Here's how the part is built. I have some questions about the finished solid (model axes, mm). Coordinates: 2 decimals unless noted, no trailing zeros. Loops run counter-clockwise (first coordinate to the right, second up) from the corner with the lowest first, then second, coordinate; pieces in that order, holes last. Notation, with made-up numbers: (42.25, 37) -> (60.25, 37) arc R35 ccw to (60.25, 72) -> close; hole circle Ø11 at (47, 52.25). An arc over 180 degrees is marked (long way). Answer as a JSON object with one key per item and string values. Group by question number.
Q1. I'm going to push a flat-ended pin straight in: pin 1 (7 mm diameter, centred on y = 29, z = 0, fed in from -X). Where does the tip first touch, or does it pass through?
Q2. Thinking about a two-plate mould opening in Y: for faces 1 (the cylindrical face through (30.12, 32.05, 0.4)), 2 (the flat face through (-1, -50, 0)), 3 (the flat face through (-35, 12, -7.5)), which applies, released by +Y, released by -Y, zero draft, split by the parting line, or undercut?
Q3. I want a section at D-D on z = 5.25. Write out the boundary of the cut face in (x, y), then the cut area to 3 significant figures.
Q4. I want a section at A-A on y = 0. Write out the boundary of the cut face in (x, z).
Q5. I want a section at B-B on x = 0. Write out the boundary of the cut face in (y, z), then the cut area to 3 significant figures.
Q6. I want a section at C-C on z = 0.5. Count the separate pieces of the cut face and the enclosed holes in it, then the cut area to 3 significant figures.
Q7. I need wall thicknesses on line 1 (Y direction, x = 0, z = 0.5); line 2 (Y direction, x = -1, z = -2.5); line 3 (Z direction, x = -27, y = 29) (3 decimals). Which ranges of each line are inside material? Lowest first, please.
```python
from build123d import *

# Parameters (mm, degrees)
SKIZZE1_W                       = 77
SKIZZE1_H                       = 100
AUFSATZ_LINEAR_AUSTRAGEN1_DEPTH = 7.5
SKIZZE2_R                       = 36.1
SCHNITT_LINEAR_AUSTRAGEN1_DEPTH = 65.863317831
SKIZZE3_R                       = 3.075
SCHNITT_LINEAR_AUSTRAGEN2_DEPTH = 93.115416734
FASE1_SIZE                      = 0.5
M3_GEWINDEBOHRUNG1_D            = 2.5


with BuildPart() as part:
    # Skizze1 → Aufsatz-Linear austragen1 (new, symmetric)
    with BuildSketch(Plane.XY):
        Rectangle(SKIZZE1_W, SKIZZE1_H)
    extrude(amount=AUFSATZ_LINEAR_AUSTRAGEN1_DEPTH, both=True)

    # Skizze2 → Schnitt-Linear austragen1 (cut, through all)
    with BuildSketch(Plane.XY.offset(7.5)):
        Circle(SKIZZE2_R)
    extrude(amount=-SCHNITT_LINEAR_AUSTRAGEN1_DEPTH, mode=Mode.SUBTRACT)

    # Skizze3 → Schnitt-Linear austragen2 (cut, through all)
    with BuildSketch(Plane(origin=(38.5, 0, 0), x_dir=(0, 0, -1), z_dir=(1, 0, 0))):
        with Locations((0, 29)):
            Circle(SKIZZE3_R)
        with Locations((0, -29)):
            Circle(SKIZZE3_R)
    extrude(amount=-SCHNITT_LINEAR_AUSTRAGEN2_DEPTH, mode=Mode.SUBTRACT)

    # Fase1
    fase1_edges = [part.edges().sort_by_distance(p)[0] for p in [
        (-36.1, 0, 7.5),
    ]]
    chamfer(fase1_edges, length=FASE1_SIZE)

    # M3 Gewindebohrung1 (through all)
    with Locations(Plane.XY.offset(7.5)):
        with Locations((-34.347488991, 20.5), (0, 40), (0, -40), (34.347488991, -20.5), (34.347488991, 20.5), (-34.347488991, -20.5)):
            Hole(M3_GEWINDEBOHRUNG1_D / 2)


solid = part.part
```
Result set:
{
 "1": {"pin 1": "stops at x = -38.5"},
 "2": {"face 1": "undercut", "face 2": "released by -Y", "face 3": "zero draft"},
 "3": {"outline": "(-38.5, -50) -> (38.5, -50) -> (38.5, 50) -> (-38.5, 50) -> close; hole circle Ø72.2 at (0, 0); hole circle Ø2.5 at (-34.35, -20.5); hole circle Ø2.5 at (-34.35, 20.5); hole circle Ø2.5 at (0, -40); hole circle Ø2.5 at (0, 40); hole circle Ø2.5 at (34.35, -20.5); hole circle Ø2.5 at (34.35, 20.5)", "area": "3,580 mm²"},
 "4": {"outline": "(-38.5, -7.5) -> (-36.1, -7.5) -> (-36.1, 7) -> (-36.6, 7.5) -> (-38.5, 7.5) -> close; (36.1, -7.5) -> (38.5, -7.5) -> (38.5, 7.5) -> (36.6, 7.5) -> (36.1, 7) -> close"},
 "5": {"outline": "(-50, -7.5) -> (-41.25, -7.5) -> (-41.25, 7.5) -> (-50, 7.5) -> close; (-38.75, -7.5) -> (-36.1, -7.5) -> (-36.1, 7) -> (-36.6, 7.5) -> (-38.75, 7.5) -> close; (36.1, -7.5) -> (38.75, -7.5) -> (38.75, 7.5) -> (36.6, 7.5) -> (36.1, 7) -> close; (41.25, -7.5) -> (50, -7.5) -> (50, 7.5) -> (41.25, 7.5) -> close", "area": "342 mm²"},
 "6": {"separate pieces": "4", "enclosed holes": "6", "area": "3,160 mm²"},
 "7": {"line 1": "y = -50 to -41.25, -38.75 to -36.1, 36.1 to 38.75, 41.25 to 50", "line 2": "y = -50 to -40.75, -39.25 to -36.09, 36.09 to 39.25, 40.75 to 50", "line 3": "z = -7.5 to -3.075, 3.075 to 7.5"}
}
